from build123d import *

# Parameters (mm, degrees)
SKETCH1_R             = 2
BOSS_EXTRUDE1_DEPTH   = 6
BOSS_EXTRUDE1_2_DEPTH = 6
SKETCH2_R             = 5.5
SKETCH2_R_2           = 4
BOSS_EXTRUDE2_DEPTH   = 6.5


with BuildPart() as part:
    # Sketch1 → Boss-Extrude1 (new body)
    with BuildSketch(Plane.XY):
        with BuildLine():
            Line((-4, 8), (-5.126415094, 1.99245283))
            ThreePointArc((-5.126415094, 1.99245283), (0, 5.5), (5.126415094, 1.99245283))
            Line((5.126415094, 1.99245283), (4, 8))
            ThreePointArc((4, 8), (0, 12), (-4, 8))
        make_face()
        with Locations((0, 8)):
            Circle(SKETCH1_R, mode=Mode.SUBTRACT)
    extrude(amount=BOSS_EXTRUDE1_DEPTH)



with BuildPart() as body_2:
    # Sketch1 → Boss-Extrude1 2 (new body)
    with BuildSketch(Plane.XY):
        with BuildLine():
            Line((-5.5, 0), (-14.456832295, -4))
            ThreePointArc((-14.456832295, -4), (0, -15), (14.456832295, -4))
            Line((14.456832295, -4), (5.5, 0))
            ThreePointArc((5.5, 0), (0, -5.5), (-5.5, 0))
        make_face()
    extrude(amount=BOSS_EXTRUDE1_2_DEPTH)


with BuildPart() as part_1:
    add(part.part)

    add(body_2.part)  # Boss-Extrude2 merges body 2
    # Sketch2 → Boss-Extrude2 (add)
    with BuildSketch(Plane.XY):
        Circle(SKETCH2_R)
        with Locations(Location((0, 0, 0), (0, 0, 180))):
            Circle(SKETCH2_R_2, mode=Mode.SUBTRACT)
    extrude(amount=BOSS_EXTRUDE2_DEPTH)

    # Sketch4 → M4 Tapped Hole1 (revolve, cut)
    with BuildSketch(Plane(origin=(0, 0, 3), x_dir=(0, 0, 1), z_dir=(1, 0, 0))):
        Polygon((0, 0), (0, 21.091420021), (1.65, 20.1), (1.65, 0), align=None)
    revolve(axis=Axis((0, 6.35, 3), (0, -1, 0)), mode=Mode.SUBTRACT)


solid = part_1.part
Build history of the part. All positions in model axes, mm. A direction names the side the tool comes from. Round coordinates to 2 decimals unless told otherwise and drop trailing zeros. Write each loop counter-clockwise with the first axis right and the second up, starting at its lowest first coordinate (ties: lowest second). Pieces come first, ordered by that corner, then holes. Notation, with made-up numbers: M 47,41 L 77,41 A5 cw 77,45 Z; hole C -14,-3 d7. An arc over 180 degrees is marked long. Answer as a JSON object with one key per item and string values. Group by question number.
(1) Cut at A-A (x = 0). Give the cut face in (y, z), and give its area (3 significant figures).
(2) Cut at D-D (x = -3.5). Give the cut face in (y, z).
(3) Which spindle directions (+Z, -Z, +X, -X, +Y, -Y) get a long thin tool onto all of the face, cutting with end or side? Do faces 4 (the cylindrical face through (5.195, 1.805, 4.198)), 5 (the flat face through (-4, -2, 6.5)), 6 (the cylindrical face through (-0.496, -9.244, 4.574)). Say none if no direction does.
(4) Flat gauge pin, fed straight in: pin 1 (3 mm diameter, centred on x = 3.5, y = -10.5, fed in from +Z). Where does the tip first touch, or does it go through?
(5) Cut at C-C (z = 3). Give the cut face in (x, y).
(6) Drill centre lines: L1, parallel to Y at x = 0, z = 5; L2, parallel to Z at x = 0, y = -10; L3, parallel to X at y = 7.5, z = 2.75. Where is each one in solid material? Low to high.
(7) Mould opens along X. For faces 1 (the flat face through (-0.2, -4.3, 0)), 2 (the flat face through (10.041, -2.028, 2.958)), 3 (the cylindrical face through (0, 10, 3)) say: pulls with the +X half, pulls with the -X half, needs draft (parallel to the pull), parting line crosses it, or undercut.
(8) Cut at B-B (y = 3). Give the cut face in (x, z).
Responses:
{
 "1": {"outline": "M -15,0 L -4,0 L -4,1.35 L -15,1.35 Z; M -15,4.65 L -4,4.65 L -4,6.5 L -5.5,6.5 L -5.5,6 L -15,6 Z; M 4,0 L 6,0 L 6,6 L 5.5,6 L 5.5,6.5 L 4,6.5 Z; M 10,0 L 12,0 L 12,6 L 10,6 Z", "area": "55.2 mm2"},
 "2": {"outline": "M -14.59,0 L -1.94,0 L -1.94,6.5 L -4.24,6.5 L -4.24,6 L -14.59,6 Z; M 1.94,0 L 9.94,0 L 9.94,6 L 4.24,6 L 4.24,6.5 L 1.94,6.5 Z"},
 "3": {"face 4": "+Z", "face 5": "+Z, +X, -X, +Y, -Y", "face 6": "-Y"},
 "4": {"pin 1": "stops at z = 6"},
 "5": {"outline": "M -14.46,-4 A15 ccw -1.65,-14.91 L -1.65,-3.64 A4 cw long 1.65,-3.64 L 1.65,-14.91 A15 ccw 14.46,-4 L 5.5,0 A5.5 ccw 5.13,1.99 L 4,8 A4 ccw -4,8 L -5.13,1.99 A5.5 ccw -5.5,0 Z; hole C 0,8 d4"},
 "6": {"L1": "y = -15 to -4, 4 to 6, 10 to 12", "L2": "z = 0 to 1.35, 4.65 to 6", "L3": "x = -4.09 to -1.94, 1.94 to 4.09"},
 "7": {"face 1": "needs draft", "face 2": "pulls with the +X half", "face 3": "undercut"},
 "8": {"outline": "M -4.94,0 L -2.65,0 L -2.65,6.5 L -4.61,6.5 L -4.61,6 L -4.94,6 Z; M 2.65,0 L 4.94,0 L 4.94,6 L 4.61,6 L 4.61,6.5 L 2.65,6.5 Z"}
}
